Source: CAD feature listing. Evaluate the final solid. Frame: model axes, mm. A direction names the side the tool comes from. Round coordinates to 2 decimals unless told otherwise and drop trailing zeros. Write each loop counter-clockwise with the first axis right and the second up, starting at its lowest first coordinate (ties: lowest second). Pieces come first, ordered by that corner, then holes.
from build123d import *

# Parameters (mm, degrees)
SKETCH2_R           = 35
BOSS_EXTRUDE1_DEPTH = 260
SKETCH3_R           = 20
CUT_EXTRUDE1_DEPTH  = 342.796723254


with BuildPart() as part:
    # Sketch1 → Revolve1 (revolve)
    with BuildSketch(Plane.XY, mode=Mode.PRIVATE) as revolve1_sk:
        Polygon((0, 135), (0, -135), (50, -135), (50, -115), (30, -115), (30, 135), align=None)
    revolve(revolve1_sk.sketch.rotate(Axis((0, 135, 0), (0, -1, 0)), 180), axis=Axis((0, 135, 0), (0, -1, 0)))

    # Sketch2 → Boss-Extrude1 (add)
    with BuildSketch(Plane(origin=(0, 0, 0), x_dir=(0, 0, 1), z_dir=(1, 0, 0))):
        with Locations(Location((0, -32.949046657, 0), (0, 0, 31.002719134))):
            Circle(SKETCH2_R)
    extrude(amount=BOSS_EXTRUDE1_DEPTH)

    # Sketch3 → Cut-Extrude1 (cut, through all)
    with BuildSketch(Plane(origin=(260, 0, 0), x_dir=(0, 0, -1), z_dir=(1, 0, 0))):
        with Locations((0, 32.949046657)):
            Circle(SKETCH3_R)
    extrude(amount=-CUT_EXTRUDE1_DEPTH, mode=Mode.SUBTRACT)


solid = part.part
1) Contact query for flat-ended pins moving along their axis: P1, Ø2.5, axis at y = 40.5, z = -32.5, coming from the -X side; P2, Ø5, axis at y = -34, z = -19.5, coming from the +X side; P3, Ø4, axis at x = 43.5, z = -28.5, coming from the +Y side. Output: stop coordinate, or through.
Taken from the geometry:
P1: stops at x = 0
P2: stops at x = 24.72
P3: stops at y = 55.81
2) Section query A-A on z = 0. Return the cut outline in (x, y), then the cut area to 3 significant figures.
Taken from the geometry:
outline: (-50, -135) - (50, -135) - (50, -115) - (30, -115) - (30, -2.05) - (260, -2.05) - (260, 12.95) - (-30, 12.95) - (-30, -115) - (-50, -115) - close; (-30, 52.95) - (260, 52.95) - (260, 67.95) - (30, 67.95) - (30, 135) - (-30, 135) - close
area: 21,500 mm2
3) Reachability of faces 4 (the face through (-47.69, -124.86, -15.02)), 5 (the face through (128.18, 66.144, 11.096)), 6 (the face through (-28.615, 11.75, -9.011)) from +Z, -Z, +X, -X, +Y, -Y: full face, straight path, thin tool, end or side. Return the list, or none.
Taken from the geometry:
face 4: -Y
face 5: +X
face 6: none
4) Section query C-C on x = 26.5. Return the cut outline in (y, z), then the cut area to 3 significant figures.
Taken from the geometry:
outline: (-135, -42.4) - (-115, -42.4) - (-115, -14.06) - (0.9, -14.06) arc R35 ccw to (65, -14.06) - (135, -14.06) - (135, 14.06) - (65, 14.06) arc R35 ccw to (0.9, 14.06) - (-115, 14.06) - (-115, 42.4) - (-135, 42.4) - close; hole circle Ø40 at (32.95, 0)
area: 9,400 mm2
5) Section query B-B on y = 47.5. Return the cut outline in (x, z), then the cut area to 3 significant figures.
Taken from the geometry:
outline: (-26.68, -13.72) arc R30 ccw to (0, -30) - (0, -31.83) - (260, -31.83) - (260, -13.72) - close; (-26.68, 13.72) - (260, 13.72) - (260, 31.83) - (0, 31.83) - (0, 30) arc R30 ccw to start
area: 10,000 mm2
6) Pull-direction query (Y, two-part tool) for faces 1 (the face through (-22, -115, 22)), 2 (the face through (-1, -135, -1)), 3 (the face through (260, 38, 21)); classes: released by +Y, released by -Y, zero draft, split by the parting line, or undercut.
Taken from the geometry:
face 1: undercut
face 2: released by -Y
face 3: zero draft
7) Material intervals for line 1 (Y direction, x = 164, z = 0); line 2 (Y direction, x = 39, z = -2), sorted ascending.
Taken from the geometry:
line 1: y = -2.05 to 12.95, 52.95 to 67.95
line 2: y = -135 to -115, -1.99 to 13.05, 52.85 to 67.89
8) Section query D-D on y = -96.5. Return the cut outline in (x, z).
Taken from the geometry:
outline: circle Ø60 at (0, 0)
